from build123d import *

# Parameters (mm, degrees)
F0_W           = 63.5
F0_H           = 38.1
F1_DEPTH       = 19.05
F3_D           = 7.14375
F3_CBORE_D     = 11.1125
F3_CBORE_DEPTH = 12.7
F5_DEPTH       = 63.501
F7_D           = 6.7564
F9_D           = 3.96875


with BuildPart() as f1:
    # F0 (on Right) → F1 (new body)
    with BuildSketch(Plane.YZ):
        with Locations((31.75, 19.05)):
            Rectangle(F0_W, F0_H)
    extrude(amount=F1_DEPTH)

    # F3 (through all)
    with Locations(Plane.YZ.offset(19.05)):
        with Locations((9.525, 19.05), (53.975, 19.05)):
            CounterBoreHole(F3_D / 2, F3_CBORE_D / 2, F3_CBORE_DEPTH)

    # F4 (on face) → F5 (cut, through all)
    with BuildSketch(Plane.XZ):
        Polygon((19.05, 38.1), (9.525, 38.1), (19.05, 0), align=None)
    extrude(amount=-F5_DEPTH, mode=Mode.SUBTRACT)

    # F7 (through all)
    with Locations(Plane(origin=(17.929412, 0, 4.482353), x_dir=(0, 1, 0), z_dir=(0.970143, 0, 0.242536))):
        with Locations((31.75, 15.015987)):
            Hole(F7_D / 2)

    # F9 (through all)
    with Locations(Plane(origin=(17.929412, 0, 4.482353), x_dir=(0, 1, 0), z_dir=(0.970143, 0, 0.242536))):
        with Locations((6.081646, 30.890987), (57.418354, 30.890987), (57.418354, -0.859013), (6.081646, -0.859013)):
            Hole(F9_D / 2)


solid = f1.part
Design review of the part built by this model. Coordinates are the model's own, in mm. A direction names the side the tool comes from. Round coordinates to 2 decimals unless told otherwise and drop trailing zeros. Order: outer loops, then holes, each group sorted by start corner. A loop starts at its lowest first (then second) coordinate and runs counter-clockwise, first axis right, second up.
1) Consider section D-D (y = 52). State the section outline as (x, z) points (3 decimals), plus the area to 3 significant figures.
The answers:
outline: (0, 0) - (19.05, 0) - (15.586, 13.857) - (6.35, 13.857) - (6.35, 16.074) - (0, 16.074) - close; (0, 22.026) - (6.35, 22.026) - (6.35, 24.243) - (12.989, 24.243) - (9.525, 38.1) - (0, 38.1) - close
area: 424 mm2
2) Clearance check with flat-ended pins moving along their axes: pin 1 Ø4 at (x, y) = (10.5, 29.5) entering from -Z; pin 2 Ø9 at (y, z) = (12, 18) entering from +X (3 decimals); pin 3 Ø6.5 at (y, z) = (53.975, 19.05) entering from -X; pin 4 Ø2 at (y, z) = (27.5, 6.5) entering from +X (3 decimals). State where each tip first meets the part, or that it passes through.
The answers:
pin 1: stops at z = 0
pin 2: stops at x = 15.675
pin 3: passes through
pin 4: stops at x = 17.675
3) Draft analysis for pull direction X (two halves, no side actions). For faces 3 (the flat face through (6.35, 54, 15)), 4 (the flat face through (9, 31, 0)), 5 (the cylindrical face through (10.563, 6.34, 3.783)), 6 (the cylindrical face through (5.322, 57.849, 31.175)), state which applies: released by +X, released by -X, zero draft, split by the parting line, or undercut.
The answers:
face 3: released by +X
face 4: zero draft
face 5: undercut
face 6: undercut
4) For L1, parallel to Y at x = 13, z = 19.05; L2, parallel to Y at x = 3.75, z = 18; L3, parallel to X at y = 13, z = 15, list the stretches that pass through material, from the lowest coordinate up.
The answers:
L1: y = 0 to 3.97, 15.08 to 28.39, 35.11 to 48.42, 59.53 to 63.5
L2: y = 0 to 6.11, 12.94 to 28.74, 34.76 to 50.56, 57.39 to 63.5
L3: x = 0 to 6.35
5) Machinability: for faces 1 (the cylindrical face through (10.042, 8.321, 13.626)), 2 (the cylindrical face through (3.131, 50.568, 20.123)), which of the approach directions +Z, -Z, +X, -X, +Y, -Y give a long, thin tool a straight path to every point of the face, cutting with its end or side? Answer none if there is none.
The answers:
face 1: +X
face 2: +X, -X
6) Consider section A-A (y = 9.5). State the section outline as (x, z) points (3 decimals), plus the area to 3 significant figures.
The answers:
outline: (0, 0) - (19.05, 0) - (15.677, 13.494) - (6.35, 13.494) - (6.35, 15.478) - (0, 15.478) - close; (0, 22.622) - (6.35, 22.622) - (6.35, 24.606) - (12.898, 24.606) - (9.525, 38.1) - (0, 38.1) - close
area: 411 mm2
7) Consider section B-B (y = 25). State the section outline as (x, z) points (3 decimals), plus the area to 3 significant figures.
The answers:
outline: (0, 0) - (19.05, 0) - (9.525, 38.1) - (0, 38.1) - close
area: 544 mm2
8) Consider section C-C (z = 33). Count the separate pieces of the cut face and the enclosed holes in it, plus the area to 3 significant figures.
The answers:
separate pieces: 3
enclosed holes: 0
area: 607 mm2
